Part model, mm, in its own coordinate system. A direction names the side the tool comes from. Give positions to 0.01 mm unless a question says otherwise; leave off trailing zeros. Order: outer loops, then holes, each group sorted by start corner. A loop starts at its lowest first (then second) coordinate and runs counter-clockwise, first axis right, second up. Notation, with made-up numbers: (21.5, 8.25) -> (30.5, 8.25) arc R23 cw to (30.5, 22.25) -> close; hole circle Ø11 at (85, 72.25). An arc over 180 degrees is marked (long way). Write item = value, one per line. Start each with the question number.
Item 1: Pull direction X, two halves, no side cores. Call faces 1 (the face through (2, 25, 8)), 2 (the face through (27, 4, 12)), 3 (the face through (55, 12, 8)): +X half, -X half, draft (parallel to the pull), parting line (faces both ways), or undercut.
Item 2: Band-saw the part on B-B on y = 22.25. Write the cut outline in (x, z).
Item 3: Band-saw the part on C-C on z = 6. Write the cut outline in (x, y).
Item 4: Tool access for faces 4 (the face through (50.5, 15, 6)), 5 (the face through (28, 3, -18.416)), 6 (the face through (28, 2, 13)), 7 (the face through (27, 20, -10)), 8 (the face through (27.64, 11.07, -19.22)): list every direction of +Z, -Z, +X, -X, +Y, -Y with a clear straight run to the whole face (end or side of a thin tool).
Item 5: Band-saw the part on D-D on z = -19. Write the cut outline in (x, y), plus the area to 3 significant figures.
Item 6: Drill centre lines: line 1 along Z through (x, y) = (25, 2.25); line 2 along X through (y, z) = (16.5, 4.5); line 3 along Z through (x, y) = (47, 4.25). Where is each one in solid material? Low to high.
Item 7: Flat gauge pins, fed straight in: P1, Ø2, axis at x = 17.5, z = -9, coming from the -Y side; P2, Ø1, axis at y = 13, z = 15.5, coming from the -X side; P3, Ø6.5, axis at x = 31.5, y = 3.5, coming from the -Z side; P4, Ø1.5, axis at x = 6, y = 7, coming from the +Z side. Where does each tip first touch, or does it go through?
Item 8: Band-saw the part on A-A on x = 25.5. Write the cut outline in (y, z).
```python
from build123d import *

# Parameters (mm, degrees)
SKETCH1_W           = 55
SKETCH1_H           = 25
BOSS_EXTRUDE1_DEPTH = 16.5
SKETCH2_W           = 46
SKETCH2_H           = 20
CUT_EXTRUDE1_DEPTH  = 14.5
SKETCH3_W           = 2.5
SKETCH3_H           = 20
CUT_EXTRUDE2_DEPTH  = 2.5
CUT_EXTRUDE3_DEPTH  = 3
CUT_EXTRUDE4_DEPTH  = 63.130910182
SKETCH8_W           = 20
SKETCH8_H           = 2
BOSS_EXTRUDE2_DEPTH = 22
SKETCH9_W           = 20
SKETCH9_H           = 2
BOSS_EXTRUDE3_DEPTH = 2
BOSS_EXTRUDE4_DEPTH = 20


with BuildPart() as part:
    # Sketch1 → Boss-Extrude1 (new body)
    with BuildSketch(Plane.XY):
        with Locations((27.5, 12.5)):
            Rectangle(SKETCH1_W, SKETCH1_H)
    extrude(amount=BOSS_EXTRUDE1_DEPTH)

    # Sketch2 → Cut-Extrude1 (cut)
    with BuildSketch(Plane.XY.offset(16.5)):
        with Locations((27.5, 15)):
            Rectangle(SKETCH2_W, SKETCH2_H)
    extrude(amount=-CUT_EXTRUDE1_DEPTH, mode=Mode.SUBTRACT)

    # Sketch3 → Cut-Extrude2 (cut)
    with BuildSketch(Plane(origin=(4.5, 0, 0), x_dir=(0, 0, -1), z_dir=(1, 0, 0))):
        with Locations((-13.25, 15)):
            Rectangle(SKETCH3_W, SKETCH3_H)
    cut_extrude2 = extrude(amount=-CUT_EXTRUDE2_DEPTH, mode=Mode.SUBTRACT)

    # Mirror1: Cut-Extrude2 across plane
    add(cut_extrude2.mirror(Plane(origin=(27.5, 0, 0), x_dir=(0, 0, 1), z_dir=(1, 0, 0))), mode=Mode.SUBTRACT)

    # Sketch4 → Cut-Extrude3 (cut)
    with BuildSketch(Plane(origin=(0, 5, 0), x_dir=(1, 0, 0), z_dir=(0, 1, 0))):
        Polygon((4.5, -12), (50.5, -12), (53, -12), (53, -14.5), (50.5, -14.5), (4.5, -14.5), (2, -14.5), (2, -12), align=None)
    extrude(amount=-CUT_EXTRUDE3_DEPTH, mode=Mode.SUBTRACT)

    # Sketch6 → Cut-Extrude4 (cut, through all)
    with BuildSketch(Plane.XY.offset(2)):
        Polygon((27.5, 20), (4.5, 20), (4.5, 25), (50.5, 25), (50.5, 20), align=None)
    extrude(amount=-CUT_EXTRUDE4_DEPTH, mode=Mode.SUBTRACT)

    # Sketch8 → Boss-Extrude2 (add)
    with BuildSketch(Plane(origin=(0, 0, 0), x_dir=(-1, 0, 0), z_dir=(0, 0, -1))):
        with Locations((-27.5, 19)):
            Rectangle(SKETCH8_W, SKETCH8_H)
    extrude(amount=BOSS_EXTRUDE2_DEPTH)

    # Sketch9 → Boss-Extrude3 (add)
    with BuildSketch(Plane.XZ.offset(-18)):
        with Locations((27.5, -21)):
            Rectangle(SKETCH9_W, SKETCH9_H)
    extrude(amount=BOSS_EXTRUDE3_DEPTH)

    # Sketch10 → Boss-Extrude4 (add)
    with BuildSketch(Plane(origin=(37.5, 0, 0), x_dir=(0, 0, -1), z_dir=(1, 0, 0))):
        Polygon((20, 16), (18.416155597, 6), (18.416155597, 0), (20.416155597, 0), (20.416155597, 6), (22, 16), align=None)
    extrude(amount=-BOSS_EXTRUDE4_DEPTH)


solid = part.part
```
Values found:
q1.face_1 = draft
q1.face_2 = undercut
q1.face_3 = +X half
q2.outline = (0, 0) -> (4.5, 0) -> (4.5, 12) -> (2, 12) -> (2, 14.5) -> (4.5, 14.5) -> (4.5, 16.5) -> (0, 16.5) -> close; (50.5, 0) -> (55, 0) -> (55, 16.5) -> (50.5, 16.5) -> (50.5, 14.5) -> (53, 14.5) -> (53, 12) -> (50.5, 12) -> close
q3.outline = (0, 0) -> (55, 0) -> (55, 25) -> (50.5, 25) -> (50.5, 5) -> (4.5, 5) -> (4.5, 25) -> (0, 25) -> close
q4.face_4 = +Z, +Y
q4.face_5 = +X, -X, -Y
q4.face_6 = +Y
q4.face_7 = +Z, -Z, +Y
q4.face_8 = +X, -X
q5.outline = (17.5, 0) -> (37.5, 0) -> (37.5, 9.69) -> (17.5, 9.69) -> close; (17.5, 18) -> (37.5, 18) -> (37.5, 20) -> (17.5, 20) -> close
q5.area = 234 mm^2
q6.line_1 = -20.42 to -18.42, 0 to 12, 14.5 to 16.5
q6.line_2 = 0 to 4.5, 50.5 to 55
q6.line_3 = 0 to 12, 14.5 to 16.5
q7.P1 = 18
q7.P2 = 0
q7.P3 = -20.53
q7.P4 = 2
q8.outline = (0, -20.42) -> (6, -20.42) -> (16, -22) -> (20, -22) -> (20, 2) -> (5, 2) -> (5, 12) -> (2, 12) -> (2, 14.5) -> (5, 14.5) -> (5, 16.5) -> (0, 16.5) -> (0, 0) -> (18, 0) -> (18, -20) -> (16, -20) -> (6, -18.42) -> (0, -18.42) -> close
